Verification items for the finished model (mm, model axes). A direction names the side the tool comes from. Coordinates: 2 decimals unless noted, no trailing zeros. Return JSON: item names as keys, results as strings. Group by question number.
Q1. Mould release check, pull along Z, two halves, no side actions. Record for faces 3 (the face through (-46.623, 6, -10)), 4 (the face through (6.278, 7.507, 26.206)), 5 (the face through (15, 6, -54.27)): pulls with the +Z half, pulls with the -Z half, needs draft (parallel to the pull), parting line crosses it, or undercut.
Q2. Section check A-A, the plane y = 9.5. Count the separate pieces of the cut face and the enclosed holes in it, then the cut area to 3 significant figures.
Q3. Go/stop test with a flat-tipped pin: pin 1 Ø5.5 at (x, z) = (6, -50.5) entering from +Y. Record where the tip stops, or that it passes through.
Q4. Thickness scan on probe 1 along Z at (x, y) = (52.5, 9); probe 2 along Z at (x, y) = (52, 12); probe 3 along X at (y, z) = (2.75, -47). Record the ranges inside material, lowest first.
Q5. Access from +Z, -Z, +X, -X, +Y, -Y to the whole of each face (thin tool, end or side, straight path). Record for faces 1 (the face through (48.68, 7.51, 27.27)), 2 (the face through (-34.023, 6.439, -49.942)).
Autodesk Inventor part; units mm, degrees
ref_plane "YZ Plane" through (0, 0, 0) normal (1, 0, 0) x (0, 1, 0)
ref_plane "XZ Plane" through (0, 0, 0) normal (0, 1, 0) x (-1, 0, 0)
ref_plane "XY Plane" through (0, 0, 0) normal (0, 0, 1) x (1, 0, 0)
sketch "Sketch1" plane through (0, 0, 0) normal (0, 1, 0) x (-1, 0, 0)
  line L0 (46.6228, 34.6302) -> (-74.0272, 34.6302)
  line L1 (-74.0272, 34.6302) -> (-74.0272, -54.2698)
  line L2 (-74.0272, -54.2698) -> (46.6228, -54.2698)
  line L3 (46.6228, -54.2698) -> (46.6228, 34.6302)
  point P0 (0, 0)
  dimension "d0" = 120.65
  dimension "d1" = 88.9
extrude "Extrusion1" add sketch "Sketch1" along normal blind 12.7
sketch "Sketch2" plane through (0, 12.7, 0) normal (0, 1, 0) x (1, 0, 0)
  line L0 (-46.6228, -34.6302) -> (74.0272, -34.6302)
  line L1 (-46.6228, 54.2698) -> (-46.6228, -34.6302)
  point P0 (0, 0)
  point P1 (6.7172, -29.5502)
  point P2 (51.1672, -29.5502)
  dimension "d4" = 0
  dimension "d5" = 5.08
  dimension "d6" = 53.34
  dimension "d7" = 44.45
hole "Hole1" at (6.7172, 12.7, 29.5502) at (51.1672, 12.7, 29.5502) direction (0, -1, 0) diameter 4.826 depth 25.4 tip angle 118 countersink diameter 9.525 countersink angle 82
sketch "Sketch3" plane through (0, 0, 0) normal (0, -1, 0) x (1, 0, 0)
  line L0 (-16.8428, 29.5502) -> (-28.8428, 29.5502)
  line L1 (-28.8428, 29.5502) -> (-28.8428, 23.5502)
  line L2 (-28.8428, 23.5502) -> (-16.8428, 23.5502)
  line L3 (-16.8428, 23.5502) -> (-16.8428, 29.5502)
  line L4 (-46.6228, 34.6302) -> (74.0272, 34.6302)
  line L5 (-46.6228, -54.2698) -> (-46.6228, 34.6302)
  point P0 (0, 0)
  dimension "d15" = 6
  dimension "d16" = 12
  dimension "d17" = 5.08
  dimension "d18" = 17.78
extrude "Extrusion2" cut sketch "Sketch3" against normal blind 1.27
sketch "Sketch4" plane through (0, 0, 0) normal (0, -1, 0) x (1, 0, 0)
  line L0 (74.0272, -54.2698) -> (-46.6228, -54.2698)
  line L1 (-28.8428, 23.5502) -> (-28.8428, 29.5502)
  line L2 (-46.6228, -54.2698) -> (-46.6228, 34.6302)
  point P0 (0, 0)
  point P1 (-32.8428, -42.0898)
  point P2 (-32.8428, -49.1898)
  point P3 (-11.9428, -49.1898)
  point P4 (-11.9428, -42.0898)
  dimension "d21" = 0
  dimension "d22" = 0
  dimension "d23" = 0
  dimension "d24" = 0
  dimension "d25" = 5.08
  dimension "d26" = 7.1
  dimension "d27" = 20.9
  dimension "d35" = 4
  dimension "d92" = 13.78
hole "Hole2" at (-32.8428, 0, -42.0898) at (-32.8428, 0, -49.1898) at (-11.9428, 0, -49.1898) at (-11.9428, 0, -42.0898) direction (0, 1, 0) diameter 2.8 depth 25.4 tip angle 118
sketch "Sketch6" plane through (0, 0, 0) normal (0, -1, 0) x (1, 0, 0)
  line L0 (-46.6228, 34.6302) -> (74.0272, 34.6302)
  line L1 (-46.6228, -54.2698) -> (-46.6228, 34.6302)
  line L2 (74.0272, -54.2698) -> (-46.6228, -54.2698)
  point P0 (0, 0)
  point P1 (69.7092, -50.0788)
  point P2 (-42.0508, -50.0788)
  point P3 (-42.0508, 30.4392)
  point P4 (69.7092, 30.4392)
  dimension "d43" = 0
  dimension "d44" = 0
  dimension "d46" = 111.76
  dimension "d47" = 0
  dimension "d48" = 0
  dimension "d50" = 4.191
  dimension "d51" = 4.572
  dimension "d91" = 4.191
hole "Hole4" at (69.7092, 0, -50.0788) at (-42.0508, 0, -50.0788) at (-42.0508, 0, 30.4392) at (69.7092, 0, 30.4392) direction (0, 1, 0) diameter 4.8 depth 25.4 tip angle 118
sketch "Sketch10" plane through (0, 12.7, 0) normal (0, 1, 0) x (1, 0, 0)
  circle A0 centre (51.1672, -29.5502) radius 2.413
  circle A1 centre (6.7172, -29.5502) radius 2.413
  line L0 (74.0272, 54.2698) -> (-46.6228, 54.2698)
  point P0 (0, 0)
  point P1 (6.7172, 49.1898)
  point P2 (51.1672, 49.1898)
  point P3 (66.6772, 28.8698)
  point P4 (-45.6228, 28.8698)
  point P5 (-46.6228, 54.2698)
  dimension "d80" = 0
  dimension "d81" = 0
  dimension "d82" = 0
  dimension "d83" = 5.08
hole "Hole7" at (6.7172, 12.7, -49.1898) at (51.1672, 12.7, -49.1898) direction (0, -1, 0) diameter 4.826 end through all countersink diameter 9.525 countersink angle 82
sketch "Sketch11" plane through (0, 0, 0) normal (0, -1, 0) x (1, 0, 0)
  line L0 (-28.8428, -3.8198) -> (-16.8428, -3.8198)
  line L1 (-16.8428, -3.8198) -> (-16.8428, -9.8198)
  line L2 (-16.8428, -9.8198) -> (-28.8428, -9.8198)
  line L3 (-28.8428, -9.8198) -> (-28.8428, -3.8198)
  line L4 (-28.8428, -43.1898) -> (-16.8428, -43.1898)
  line L5 (-16.8428, -43.1898) -> (-16.8428, -49.1898)
  line L6 (-16.8428, -49.1898) -> (-28.8428, -49.1898)
  line L7 (-28.8428, -49.1898) -> (-28.8428, -43.1898)
  line L8 (-28.8428, 23.5502) -> (-28.8428, 29.5502)
  line L9 (-16.8428, 29.5502) -> (-16.8428, 23.5502)
  line L10 (74.0272, -54.2698) -> (-46.6228, -54.2698)
  point P0 (0, 0)
  dimension "d93" = 0
  dimension "d94" = 0
  dimension "d95" = 0
  dimension "d96" = 0
  dimension "d97" = 6
  dimension "d98" = 6
  dimension "d99" = 5.08
  dimension "d100" = 44.45
extrude "Extrusion4" cut sketch "Sketch11" against normal blind 1.27
sketch "Sketch12" plane through (0, 0, 0) normal (0, -1, 0) x (1, 0, 0)
  circle A0 centre (-42.0508, 30.4392) radius 2.4
  circle A1 centre (69.7092, 30.4392) radius 2.4
  circle A2 centre (69.7092, -50.0788) radius 2.4
  circle A3 centre (-42.0508, -50.0788) radius 2.4
  point P0 (0, 0)
hole "Hole8" at (-42.0508, 0, 30.4392) at (69.7092, 0, 30.4392) at (69.7092, 0, -50.0788) at (-42.0508, 0, -50.0788) direction (0, 1, 0) diameter 4.826 end through all
sketch "Sketch13" plane through (0, 0, 0) normal (0, -1, 0) x (1, 0, 0)
  circle A0 centre (-32.8428, -42.0898) radius 1.4
  circle A1 centre (-32.8428, -49.1898) radius 1.4
  line L0 (-46.6228, 34.6302) -> (74.0272, 34.6302)
  circle A2 centre (-11.9428, -42.0898) radius 1.4
  point P0 (0, 0)
  point P1 (-32.8428, -10.3398)
  point P2 (-32.8428, -3.2278)
  point P3 (-32.8428, 22.9462)
  point P4 (-32.8428, 30.0582)
  point P5 (-39.7887, 34.6302)
  point P6 (67.4471, 34.6302)
  point P7 (-11.9428, -10.3398)
  point P8 (-11.9428, -3.2278)
  point P9 (-11.9428, 22.9462)
  point P10 (-11.9428, 30.0582)
  dimension "d110" = 0
  dimension "d111" = 0
  dimension "d112" = 0
  dimension "d113" = 7.112
  dimension "d114" = 7.112
  dimension "d115" = 31.75
  dimension "d116" = 4.572
  dimension "d117" = 0
  dimension "d118" = 0
  dimension "d119" = 0
  dimension "d120" = 0
  dimension "d121" = 0
  dimension "d122" = 0
  dimension "d123" = 0
  dimension "d124" = 0
hole "Hole9" at (-32.8428, 0, -10.3398) at (-32.8428, 0, -3.2278) at (-32.8428, 0, 22.9462) at (-32.8428, 0, 30.0582) at (-11.9428, 0, -10.3398) at (-11.9428, 0, -3.2278) at (-11.9428, 0, 22.9462) at (-11.9428, 0, 30.0582) direction (0, 1, 0) diameter 2.8 end through all
sketch "Sketch15" plane through (0, 12.7, 0) normal (0, 1, 0) x (1, 0, 0)
  circle A0 centre (6.7172, 49.1898) radius 2.413
  circle A1 centre (51.1672, 49.1898) radius 2.413
  circle A2 centre (6.7172, -29.5502) radius 2.413
  circle A3 centre (51.1672, -29.5502) radius 2.413
  circle A4 centre (6.7172, 49.1898) radius 3.3734
  circle A5 centre (6.7172, -29.5502) radius 3.3734
  circle A6 centre (51.1672, -29.5502) radius 3.3734
  circle A7 centre (51.1672, 49.1898) radius 3.3734
  point P0 (0, 0)
  dimension "d138" = 6.7469
  dimension "d139" = 6.7469
  dimension "d140" = 6.7469
  dimension "d141" = 6.7469
extrude "Extrusion6" cut sketch "Sketch15" against normal blind 8.89
equation "\"d15\" = CanConPinWidth"
equation "\"d16\" = CanConPinLength"
equation "\"d28\" = CanConHoleDiam"
equation "\"d52\" = LegoMainHole"
equation "\"d125\" = CanConHoleDiam"
equation "\"LegoMainHole\" = 4.8"
equation "\"TalonSRXWidth\" = 31.75"
equation "\"TalonSRXFromSide\" = 15.875"
equation "\"TalonSRXBetweenHoles\" = 50.8"
equation "\"CanConPinWidth\" = 6"
equation "\"CanConPinLength\" = 12"
equation "\"CanConBetweenSideHoles\" = 20.9"
equation "\"CanConBetweenTopHoles\" = 7.1"
equation "\"CanConHoleDiam\" = 2.8"
equation "\"CanConHoleFromTopPin\" = 4"
properties part number "SparkMaxPlate"
Numbers:
{
 "1": {"face 3": "needs draft", "face 4": "undercut", "face 5": "pulls with the -Z half"},
 "2": {"separate pieces": "1", "enclosed holes": "20", "area": "10,400 mm2"},
 "3": {"pin 1": "stops at y = 12.1"},
 "4": {"probe 1": "z = -54.27 to -52.29, -46.09 to 26.45, 32.65 to 34.63", "probe 2": "z = -54.27 to -53.26, -45.12 to 25.48, 33.62 to 34.63", "probe 3": "x = -46.62 to 5.7, 7.73 to 50.15, 52.18 to 74.03"},
 "5": {"face 1": "+Y", "face 2": "+Y, -Y"}
}
